```python
from build123d import *

# Parameters (mm, degrees)
F0_W     = 55
F0_H     = 85
F1_DEPTH = 35
F3_T     = -2.5
F4_R     = 5
F5_DEPTH = 25


# Not quite as in the source:
# - the program builds the solid bodies; features that only make, move or delete a surface that nothing else refers to are left out


with BuildPart() as f1:
    # F0 (on Top) → F1 (new body)
    with BuildSketch(Plane.XY):
        with Locations((-28.1140384175, 11.1121237278)):
            Rectangle(F0_W, F0_H)
    extrude(amount=F1_DEPTH)

    # F3
    f3_openings = [f1.faces().sort_by_distance(p)[0] for p in [
        (-28.114038, 11.112124, 0),
    ]]
    offset(amount=F3_T, openings=f3_openings)

    # F4 (on face) → F5 (cut)
    with BuildSketch(Plane.YZ.offset(-0.6140384175)):
        with Locations((-1.3878762722, 20)):
            Circle(F4_R)
    extrude(amount=-F5_DEPTH, mode=Mode.SUBTRACT)


solid = f1.part
```
Could you check a few things on this model? Use its own coordinates, in mm. A direction names the side the tool comes from. Give positions to 0.01 mm unless a question says otherwise; leave off trailing zeros. Write each loop counter-clockwise with the first axis right and the second up, starting at its lowest first coordinate (ties: lowest second). Pieces come first, ordered by that corner, then holes. Notation, with made-up numbers: (88, 25.5) -> (97, 25.5) arc R24 ccw to (97, 61.5) -> close; hole circle Ø4 at (76.25, -4). An arc over 180 degrees is marked (long way). Write each question's results on one line, items separated by ' | '.
1. If we mould it in two halves opening along X, with no side actions, what happens to faces 4 (the flat face through (-3.114, 11, 16)), 5 (the flat face through (-0.614, 11, 17)), 6 (the flat face through (-55.614, 11, 17))? For each: released by +X, released by -X, zero draft, split by the parting line, or undercut.
Check sheet entries:
face 4: undercut | face 5: released by +X | face 6: released by -X
2. I want a section at B-B, the plane x = -46.5. Write out the boundary of the cut face in (y, z).
Check sheet entries:
outline: (-31.39, 0) -> (-28.89, 0) -> (-28.89, 32.5) -> (51.11, 32.5) -> (51.11, 0) -> (53.61, 0) -> (53.61, 35) -> (-31.39, 35) -> close
3. I want a section at C-C, the plane y = -1.5. Write out the boundary of the cut face in (x, z).
Check sheet entries:
outline: (-55.61, 0) -> (-53.11, 0) -> (-53.11, 32.5) -> (-3.11, 32.5) -> (-3.11, 25) -> (-0.61, 25) -> (-0.61, 35) -> (-55.61, 35) -> close; (-3.11, 0) -> (-0.61, 0) -> (-0.61, 15) -> (-3.11, 15) -> close
4. Will this pin go through, and if not, where does the flat tip stop? pin 1 Ø10 at (x, y) = (-13.5, -9.5) entering from -Z.
Check sheet entries:
pin 1: stops at z = 32.5
5. On a 3-axis mill with a long thin cutter (end or side, diameter ignored), from which of +Z, -Z, +X, -X, +Y, -Y can I reach the whole of each face in a straight line? I mean faces 1 (the flat face through (-28, 12, 35)), 2 (the cylindrical face through (-1.85, -2.47, 15.12)), 3 (the flat face through (-28, -28.888, 16)). Say none if no direction works.
Check sheet entries:
face 1: +Z, +X, -X, +Y, -Y | face 2: +X | face 3: -Z
6. I want a section at D-D, the plane y = 13. Write out the boundary of the cut face in (x, z), then the cut area to 3 significant figures.
Check sheet entries:
outline: (-55.61, 0) -> (-53.11, 0) -> (-53.11, 32.5) -> (-3.11, 32.5) -> (-3.11, 0) -> (-0.61, 0) -> (-0.61, 35) -> (-55.61, 35) -> close | area: 300 mm²
7. I need wall thicknesses on L1, parallel to X at y = 18, z = 20; L2, parallel to Y at x = -14.5, z = 23; L3, parallel to X at y = -5, z = 20. Which ranges of each line are inside material? Lowest first, please.
Check sheet entries:
L1: x = -55.61 to -53.11, -3.11 to -0.61 | L2: y = -31.39 to -28.89, 51.11 to 53.61 | L3: x = -55.61 to -53.11
8. I want a section at A-A, the plane z = 7.5. Write out the boundary of the cut face in (x, y), then the cut area to 3 significant figures.
Check sheet entries:
outline: (-55.61, -31.39) -> (-0.61, -31.39) -> (-0.61, 53.61) -> (-55.61, 53.61) -> close; hole (-53.11, -28.89) -> (-3.11, -28.89) -> (-3.11, 51.11) -> (-53.11, 51.11) -> close | area: 675 mm²
